Model file for the job. Use its own axes, mm. Round coordinates to 2 decimals unless told otherwise and drop trailing zeros. Loops run counter-clockwise (first coordinate to the right, second up) from the corner with the lowest first, then second, coordinate; pieces in that order, holes last. Notation, with made-up numbers: (-30, 12) -> (-20, 12) arc R21 cw to (-20, 18) -> close; hole circle Ø10 at (-12, 4.25). An arc over 180 degrees is marked (long way). Use a Markdown table: item, result. Add a question column.
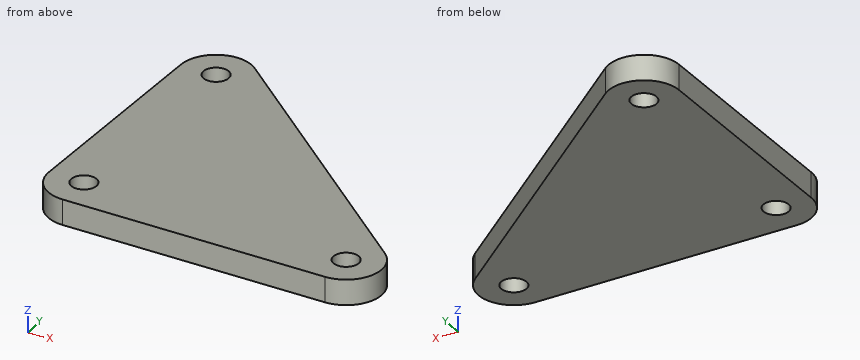
```python
from build123d import *

# Parameters (mm, degrees)
SKETCH1_R           = 3.175
BOSS_EXTRUDE1_DEPTH = 6.35
FILLET1_R           = 8.89


with BuildPart() as part:
    # Sketch1 → Boss-Extrude1 (new body)
    with BuildSketch(Plane.XY):
        Polygon((-9.141712801, -8.592188489), (-6.721283646, 75.262377261), (90.721451865, -11.8986691), align=None)
        with Locations((1.612954285, 55.88)):
            Circle(SKETCH1_R, mode=Mode.SUBTRACT)
        Circle(SKETCH1_R, mode=Mode.SUBTRACT)
        with Locations((66.548, -2.203411763)):
            Circle(SKETCH1_R, mode=Mode.SUBTRACT)
    extrude(amount=BOSS_EXTRUDE1_DEPTH)

    # Fillet1
    fillet1_edges = [part.edges().sort_by_distance(p)[0] for p in [
        (-9.141712801, -8.592188489, 3.175),
        (-6.721283646, 75.262377261, 3.175),
        (90.721451865, -11.8986691, 3.175),
    ]]
    fillet(fillet1_edges, radius=FILLET1_R)


solid = part.part
```
1) Wall check: probe 1 along Y at (x, z) = (-0.5, 5.75); probe 2 along X at (y, z) = (57, 2.5); probe 3 along X at (y, z) = (16, 4.5). Give the ranges that are in metal, low to high. Write a range as from..to.
2) Cut at A-A on z = 2.25. Count the separate pieces of the cut face and the enclosed holes in it, and give its area (3 significant figures).
3) Cut at B-B on y = 37. Write the cut outline in (x, z).
4) Pin check, flat tips, straight feed: pin 1 Ø1.5 at (y, z) = (26, 4) entering from -X; pin 2 Ø3 at (x, z) = (28.5, 2.5) entering from +Y. Stop position of each tip, or through.
5) Cut at C-C on x = 9. Write the cut outline in (y, z).
Established:
| question | item | result |
|---|---|---|
| 1 | probe 1 | y = -8.88..-3.14, 3.14..53.51, 58.25..64.52 |
| 1 | probe 2 | x = -7.21..-1.36, 4.58..13.7 |
| 1 | probe 3 | x = -8.43..59.53 |
| 2 | separate pieces | 1 |
| 2 | enclosed holes | 3 |
| 2 | area | 3,880 mm^2 |
| 3 | outline | (-7.83, 0) -> (36.05, 0) -> (36.05, 6.35) -> (-7.83, 6.35) -> close |
| 4 | pin 1 | stops at x = -8.16 |
| 4 | pin 2 | stops at y = 45.1 |
| 5 | outline | (-9.19, 0) -> (61.2, 0) -> (61.2, 6.35) -> (-9.19, 6.35) -> close |
